Verification items for this drawing (mm, ordinates from the low corner). Round coordinates to 2 decimals unless told otherwise and drop trailing zeros. Order: outer loops, then holes, each group sorted by start corner. A loop starts at its lowest first (then second) coordinate and runs counter-clockwise, first axis right, second up. Notation, with made-up numbers: (-3.5, 79.25) -> (32.5, 79.25) arc R21 cw to (32.5, 102.25) -> close; hole circle Ø4 at (54.25, -20.75). An arc over 180 degrees is marked (long way). Answer in a Markdown table with one row per item.
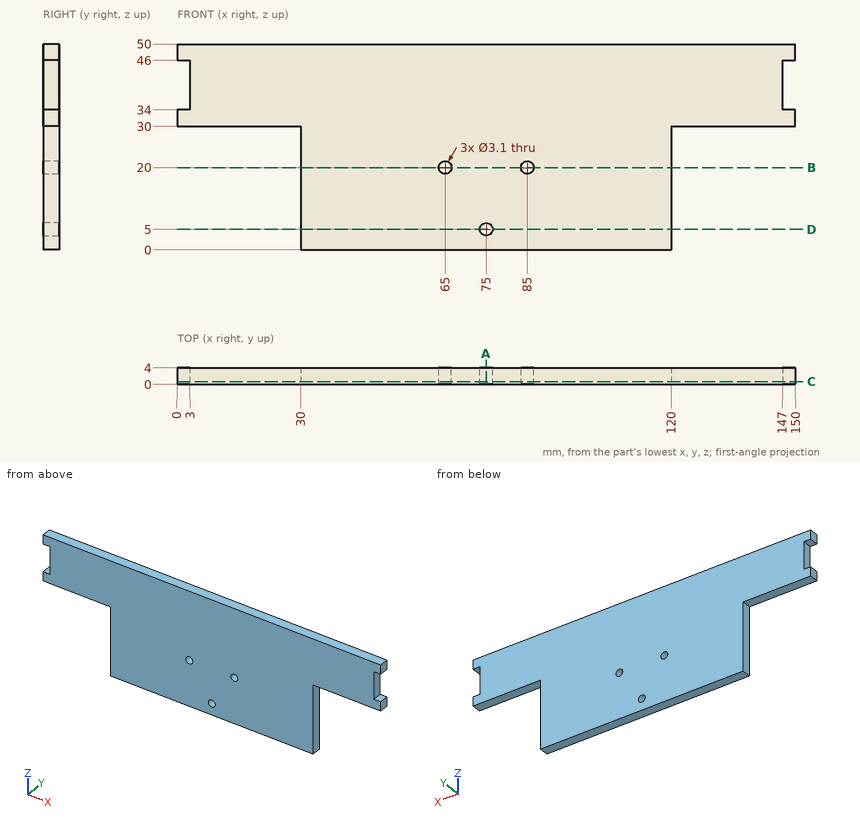
Item 1: Cross-section at C-C (y = 0.65). Record the boundary of the cut face in (x, z).
Result sheet:
| item | result |
|---|---|
| outline | (0, 30) -> (30, 30) -> (30, 0) -> (120, 0) -> (120, 30) -> (150, 30) -> (150, 34) -> (147, 34) -> (147, 46) -> (150, 46) -> (150, 50) -> (0, 50) -> (0, 46) -> (3, 46) -> (3, 34) -> (0, 34) -> close; hole circle Ø3.1 at (65, 20); hole circle Ø3.1 at (75, 5); hole circle Ø3.1 at (85, 20) |
Item 2: Depth check by flat-ended pin: P1, Ø2, axis at x = 140.5, y = 2.5, coming from the -Z side; P2, Ø1.2, axis at y = 3, z = 39.5, coming from the +X side; P3, Ø1.2, axis at y = 2.5, z = 21, coming from the -X side. Enter the tip coordinate at first touch or a pass-through.
Result sheet:
| item | result |
|---|---|
| P1 | stops at z = 30 |
| P2 | stops at x = 147 |
| P3 | stops at x = 30 |
Item 3: Cross-section at B-B (z = 20). Record the boundary of the cut face in (x, y), and give its area (3 significant figures).
Result sheet:
| item | result |
|---|---|
| outline | (30, 0) -> (63.45, 0) -> (63.45, 4) -> (30, 4) -> close; (66.55, 0) -> (83.45, 0) -> (83.45, 4) -> (66.55, 4) -> close; (86.55, 0) -> (120, 0) -> (120, 4) -> (86.55, 4) -> close |
| area | 335 mm^2 |
Item 4: Scan lines: line 1 (X direction, y = 1.1, z = 20); line 2 (Z direction, x = 85, y = 2.75); line 3 (X direction, y = 1.85, z = 5). Record each from-to range of solid material in increasing order. Write a range as [from, to].
Result sheet:
| item | result |
|---|---|
| line 1 | x = [30, 63.45], [66.55, 83.45], [86.55, 120] |
| line 2 | z = [0, 18.45], [21.55, 50] |
| line 3 | x = [30, 73.45], [76.55, 120] |
Item 5: Cross-section at A-A (x = 75). Record the boundary of the cut face in (y, z), and give its area (3 significant figures).
Result sheet:
| item | result |
|---|---|
| outline | (0, 0) -> (4, 0) -> (4, 3.45) -> (0, 3.45) -> close; (0, 6.55) -> (4, 6.55) -> (4, 50) -> (0, 50) -> close |
| area | 188 mm^2 |
Item 6: Cross-section at D-D (z = 5). Record the boundary of the cut face in (x, y).
Result sheet:
| item | result |
|---|---|
| outline | (30, 0) -> (73.45, 0) -> (73.45, 4) -> (30, 4) -> close; (76.55, 0) -> (120, 0) -> (120, 4) -> (76.55, 4) -> close |
